from build123d import *

# Parameters (mm, degrees)
SKETCH1_W           = 40
SKETCH1_H           = 110
BOSS_EXTRUDE1_DEPTH = 17
SKETCH4_W           = 110
SKETCH4_H           = 75
BOSS_EXTRUDE2_DEPTH = 10
SKETCH5_W           = 15
SKETCH5_H           = 50
CUT_EXTRUDE1_DEPTH  = 17
SKETCH6_R           = 4.6
CUT_EXTRUDE2_DEPTH  = 10
FILLET1_R           = 30
FILLET2_R           = 3
FILLET3_R           = 5
FILLET4_R           = 2


with BuildPart() as part:
    # Sketch1 → Boss-Extrude1 (new body)
    with BuildSketch(Plane(origin=(0, 0, 0), x_dir=(1, 0, 0), z_dir=(0, 1, 0))):
        with Locations((20, 55)):
            Rectangle(SKETCH1_W, SKETCH1_H)
    extrude(amount=BOSS_EXTRUDE1_DEPTH)

    # Sketch4 → Boss-Extrude2 (add)
    with BuildSketch(Plane(origin=(0, 0, 0), x_dir=(0, 0, -1), z_dir=(1, 0, 0))):
        with Locations((55, 54.5)):
            Rectangle(SKETCH4_W, SKETCH4_H)
    extrude(amount=BOSS_EXTRUDE2_DEPTH)

    # Sketch5 → Cut-Extrude1 (cut)
    with BuildSketch(Plane(origin=(0, 17, 0), x_dir=(1, 0, 0), z_dir=(0, 1, 0))):
        with Locations((25, 55)):
            Rectangle(SKETCH5_W, SKETCH5_H)
    extrude(amount=-CUT_EXTRUDE1_DEPTH, mode=Mode.SUBTRACT)

    # Sketch6 → Cut-Extrude2 (cut)
    with BuildSketch(Plane(origin=(10, 0, 0), x_dir=(0, 0, -1), z_dir=(1, 0, 0))):
        with Locations((55, 54.7)):
            Circle(SKETCH6_R)
    extrude(amount=-CUT_EXTRUDE2_DEPTH, mode=Mode.SUBTRACT)

    # Fillet1
    fillet1_edges = [part.edges().sort_by_distance(p)[0] for p in [
        (5, 92, 0),
        (5, 92, -110),
    ]]
    fillet(fillet1_edges, radius=FILLET1_R)

    # Fillet2
    fillet2_edges = [part.edges().sort_by_distance(p)[0] for p in [
        (0, 31, 0),
        (0, 92, -55),
        (0, 31, -110),
        (0, 83.213203436, -101.213203436),
        (0, 83.213203436, -8.786796564),
    ]]
    fillet(fillet2_edges, radius=FILLET2_R)

    # Fillet3
    fillet3_edges = [part.edges().sort_by_distance(p)[0] for p in [
        (10, 17, -55),
    ]]
    fillet(fillet3_edges, radius=FILLET3_R)

    # Fillet4
    fillet4_edges = [part.edges().sort_by_distance(p)[0] for p in [
        (40, 17, -55),
        (40, 0, -55),
        (40, 8.5, -110),
        (40, 8.5, 0),
    ]]
    fillet(fillet4_edges, radius=FILLET4_R)


solid = part.part
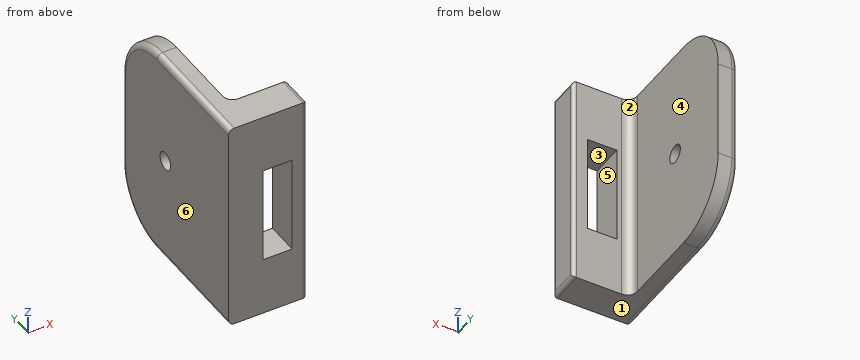
Could you check a few things on this model? Use its own coordinates, in mm. Face numbers are marked on the shaded views. A direction names the side the tool comes from. Give positions to 0.01 mm unless a question says otherwise; leave off trailing zeros. Loops run counter-clockwise (first coordinate to the right, second up) from the corner with the lowest first, then second, coordinate; pieces in that order, holes last. Notation, with made-up numbers: (39.5, 19.25) -> (51.5, 19.25) arc R18 cw to (51.5, 32.25) -> close; hole circle Ø6 at (25.5, 69). An arc over 180 degrees is marked (long way). Answer as CSV lines item,"result". Start each with the question number.
(1) We'd pull the mould along Z, two halves only. Please class the marked faces 1, 2 and 3: released by +Z, released by -Z, zero draft, split by the parting line, or undercut.
(2) I need wall thicknesses on probe 1 along Z at (x, y) = (24, 5.5); probe 2 along Y at (x, z) = (3, -55); probe 3 along X at (y, z) = (25.5, -95.5). Which ranges of each line are inside material? Lowest first, please.
(3) If we section it at A-A on y = 54.7: Write out the boundary of the cut face in (x, z).
(4) If we section it at B-B on z = -33: Write out the boundary of the cut face in (x, y).
(5) Which directions (+Z, -Z, +X, -X, +Y, -Y) give clear straight access to the entire face, cutting with the end or side of a thin tool? Please do the marked faces 4, 5 and 6.
(6) If we section it at C-C on x = 21: Write out the boundary of the cut face in (y, z).
(7) If we section it at D-D on z = -55: Write out the boundary of the cut face in (x, y).
(8) I'm going to push flat-ended pins straight in: pin 1 Ø1 at (x, z) = (13.5, -85.5) entering from +Y; pin 2 Ø12 at (y, z) = (54.7, -55) entering from +X; pin 3 Ø5 at (x, z) = (12, -87) entering from +Y. Where does each tip first touch, or does it pass through?
Computed:
1,face 1,"released by -Z"
1,face 2,"zero draft"
1,face 3,"undercut"
2,probe 1,"z = -110 to -80, -30 to 0"
2,probe 2,"y = 0 to 50.1, 59.3 to 92"
2,probe 3,"x = 0 to 10"
3,outline,"(0, -107) arc R3 ccw to (3, -110) -> (10, -110) -> (10, -59.6) -> (0, -59.6) -> close; (0, -50.4) -> (10, -50.4) -> (10, 0) -> (3, 0) arc R3 ccw to (0, -3) -> close"
4,outline,"(0, 0) -> (17.5, 0) -> (17.5, 17) -> (15, 17) arc R5 cw to (10, 22) -> (10, 92) -> (3, 92) arc R3 ccw to (0, 89) -> close; (32.5, 0) -> (38, 0) arc R2 ccw to (40, 2) -> (40, 15) arc R2 ccw to (38, 17) -> (32.5, 17) -> close"
5,face 4,"+Z, -Z, +X, +Y"
5,face 5,"+Y, -Y"
5,face 6,"+Z, -Z, -X, +Y, -Y"
6,outline,"(0, -110) -> (17, -110) -> (17, -80) -> (0, -80) -> close; (0, -30) -> (17, -30) -> (17, 0) -> (0, 0) -> close"
7,outline,"(0, 0) -> (17.5, 0) -> (17.5, 17) -> (15, 17) arc R5 cw to (10, 22) -> (10, 50.1) -> (0, 50.1) -> close; (0, 59.3) -> (10, 59.3) -> (10, 92) -> (3, 92) arc R3 ccw to (0, 89) -> close; (32.5, 0) -> (38, 0) arc R2 ccw to (40, 2) -> (40, 15) arc R2 ccw to (38, 17) -> (32.5, 17) -> close"
8,pin 1,"stops at y = 17.42"
8,pin 2,"stops at x = 10"
8,pin 3,"stops at y = 91.49"
